Geometry check sheet. Reference: the model listing, model coordinates, mm. Face numbers are marked on the shaded views. A direction names the side the tool comes from. Coordinates: 2 decimals unless noted, no trailing zeros. Write each loop counter-clockwise with the first axis right and the second up, starting at its lowest first coordinate (ties: lowest second). Pieces come first, ordered by that corner, then holes. Notation, with made-up numbers: (0.25, 21) -> (7.25, 21) arc R11 cw to (7.25, 29) -> close; hole circle Ø10 at (-2, 77.25). An arc over 180 degrees is marked (long way). Put each result on its own line as item: value. Start each with the question number.
from build123d import *

# Parameters (mm, degrees)
SKETCH1_R               = 4
FEMALE_SHAFT_DEPTH      = 5
SKETCH6_W               = 3
SKETCH6_H               = 15
MALE_START              = -8
MALE_SHAFT_INSERT_DEPTH = 16
CHAMFER1_SIZE           = 0.45
SKETCH7_R               = 1
BOSS_EXTRUDE1_DEPTH     = 4


# Read off the part's stored shape, not the designer's step: Male Shaft Insert
with BuildPart() as part:
    # Sketch1 → Female Shaft (new, symmetric)
    with BuildSketch(Plane(origin=(0, 0, 0), x_dir=(0, 0, -1), z_dir=(1, 0, 0))):
        Circle(SKETCH1_R)
        with BuildLine():
            Line((-1.260952021, 2.5), (1.260952021, 2.5))
            ThreePointArc((1.260952021, 2.5), (0, -2.8), (-1.260952021, 2.5))
        make_face(mode=Mode.SUBTRACT)
    extrude(amount=FEMALE_SHAFT_DEPTH, both=True)

    # Sketch6 → Spool Edge (revolve)
    with BuildSketch(Plane.XY, mode=Mode.PRIVATE) as spool_edge_sk:
        with Locations((6.5, 7.5)):
            Rectangle(SKETCH6_W, SKETCH6_H)
    spool_edge = revolve(spool_edge_sk.sketch.rotate(Axis((0, 0, 0), (1, 0, 0)), 90), axis=Axis((0, 0, 0), (1, 0, 0)))

    # Spool Edge Mirror: Spool Edge across plane
    add(spool_edge.mirror(Plane(origin=(0, 0, 0), x_dir=(0, 0, 1), z_dir=(1, 0, 0))))

    # Male Shaft Insert outline → Male Shaft Insert (cut)
    with BuildSketch(Plane(origin=(0, 0, 0), x_dir=(0, 0, -1), z_dir=(1, 0, 0)).offset(MALE_START)):
        with BuildLine():
            Line((1.260952021, 2.5), (-1.260952021, 2.5))
            ThreePointArc((-1.260952021, 2.5), (0, -2.8), (1.260952021, 2.5))
        make_face()
    extrude(amount=MALE_SHAFT_INSERT_DEPTH, mode=Mode.SUBTRACT)

    # Chamfer1
    chamfer1_edges = [part.edges().sort_by_distance(p)[0] for p in [
        (8, 2.5, 0),
        (8, -2.8, 0),
    ]]
    chamfer(chamfer1_edges, length=CHAMFER1_SIZE)

    # Sketch7 → Boss-Extrude1 (add)
    with BuildSketch(Plane.ZY.offset(8)):
        with Locations((0, 12.433518361)):
            Circle(SKETCH7_R)
    extrude(amount=BOSS_EXTRUDE1_DEPTH)


solid = part.part
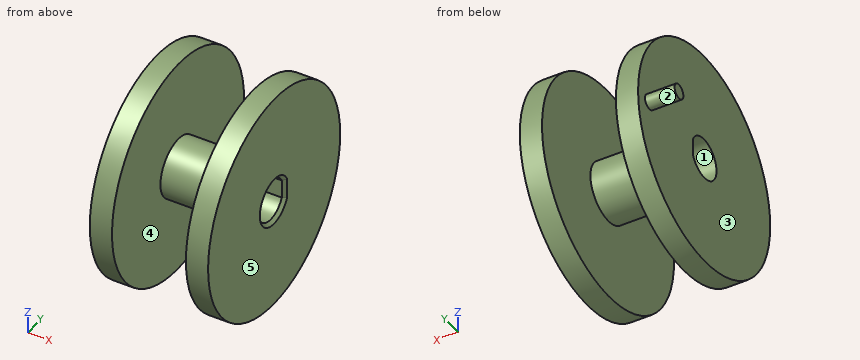
Item 1: Access from +Z, -Z, +X, -X, +Y, -Y to the whole of each face (thin tool, end or side, straight path). Record for the marked faces 4 and 5.
Item 2: Mould release check, pull along Y, two halves, no side actions. Record for the marked faces 1, 2 and 3: released by +Y, released by -Y, zero draft, split by the parting line, or undercut.
Item 3: Section check A-A, the plane z = 0. Enter the section's corners in (x, y), and give its area (3 significant figures).
Item 4: Go/stop test with flat-tipped pins: P1, Ø1.5, axis at y = -1.5, z = -4.5, coming from the -X side; P2, Ø1.5, axis at x = 1.5, y = -1.5, coming from the -Z side; P3, Ø4, axis at x = 1, z = 4.5, coming from the +Y side; P4, Ø3.5, axis at y = 0, z = 0, coming from the -X side. Record where each tip stops, or that it passes through.
Item 5: Section check B-B, the plane y = 0. Enter the section's corners in (x, z), and give its area (3 significant figures).
Item 6: Scan lines: line 1 along X through (y, z) = (-13.5, -2.5); line 2 along Y through (x, z) = (4.25, 0); line 3 along Y through (x, z) = (5.75, 0). Record each from-to range of solid material in increasing order. Write a range as [from, to].
Item 7: Section check C-C, the plane z = -9. Enter the section's corners in (x, y).
From the geometry:
1. face 4: none
1. face 5: +Z, -Z, +X, +Y, -Y
2. face 1: undercut
2. face 2: split by the parting line
2. face 3: zero draft
3. outline: (-12, 11.43) -> (-8, 11.43) -> (-8, 2.5) -> (7.55, 2.5) -> (8, 2.95) -> (8, 15) -> (5, 15) -> (5, 4) -> (-5, 4) -> (-5, 15) -> (-8, 15) -> (-8, 13.43) -> (-12, 13.43) -> close; (-8, -15) -> (-5, -15) -> (-5, -4) -> (5, -4) -> (5, -15) -> (8, -15) -> (8, -3.25) -> (7.55, -2.8) -> (-8, -2.8) -> close
3. area: 183 mm²
4. P1: x = -8
4. P2: z = -3.93
4. P3: y = 3.12
4. P4: through
5. outline: (-8, -15) -> (-5, -15) -> (-5, -4) -> (5, -4) -> (5, -15) -> (8, -15) -> (8, -3.25) -> (7.55, -2.8) -> (-8, -2.8) -> close; (-8, 2.8) -> (7.55, 2.8) -> (8, 3.25) -> (8, 15) -> (5, 15) -> (5, 4) -> (-5, 4) -> (-5, 15) -> (-8, 15) -> close
5. area: 170 mm²
6. line 1: [-8, -5], [5, 8]
6. line 2: [-4, -2.8], [2.5, 4]
6. line 3: [-15, -2.8], [2.5, 15]
7. outline: (-8, -12) -> (-5, -12) -> (-5, 12) -> (-8, 12) -> close; (5, -12) -> (8, -12) -> (8, 12) -> (5, 12) -> close
